from build123d import *

# Parameters (mm, degrees)
F0_W     = 30
F0_H     = 12
F1_DEPTH = 4.5
F2_W     = 30
F2_H     = 12
F3_DEPTH = 30


with BuildPart() as f1:
    # F0 (on Front) → F1 (new body, symmetric)
    with BuildSketch(Plane.XZ):
        with BuildLine():
            Line((8.60261, 24.451202), (-2.39739, 24.451202))
            ThreePointArc((-2.39739, 24.451202), (-9.114904, 21.668717), (-11.89739, 14.951202))
            Line((-11.89739, 14.951202), (-11.89739, -3.548798))
            Line((-11.89739, -3.548798), (18.10261, -3.548798))
            Line((18.10261, -3.548798), (18.10261, 14.951202))
            ThreePointArc((18.10261, 14.951202), (15.320125, 21.668717), (8.60261, 24.451202))
        make_face()
        with Locations((3.10261, -9.548798)):
            Rectangle(F0_W, F0_H)
    extrude(amount=F1_DEPTH, both=True)

    # F2 (on Front) → F3 (join)
    with BuildSketch(Plane.XZ):
        with Locations((3.045083, -9.593663)):
            Rectangle(F2_W, F2_H)
    extrude(amount=F3_DEPTH)


solid = f1.part
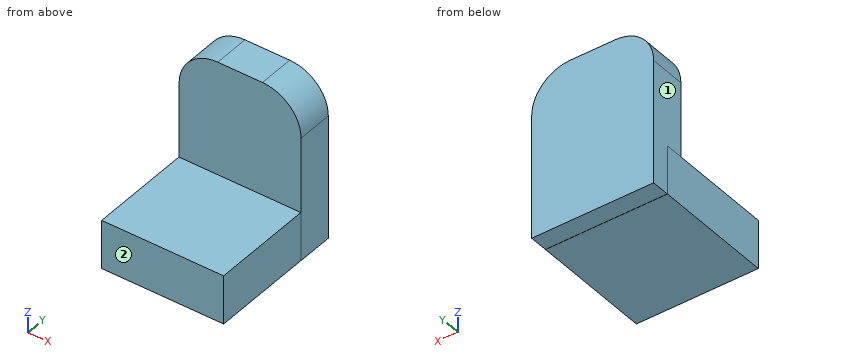
Verification items for the finished model (mm, model axes). Face numbers are marked on the shaded views. A direction names the side the tool comes from. Round coordinates to 2 decimals unless told otherwise and drop trailing zeros. Loops run counter-clockwise (first coordinate to the right, second up) from the corner with the lowest first, then second, coordinate; pieces in that order, holes last. Notation, with made-up numbers: (75.25, 45.25) - (90.25, 45.25) arc R16 cw to (90.25, 61.25) - close; hole circle Ø5 at (71, -19). An arc over 180 degrees is marked (long way). Answer in a Markdown table with one row per item. Add a question column.
Q1. Tool access check on the marked faces 1 and 2. Record the directions out of +Z, -Z, +X, -X, +Y, -Y that give a thin tool (end or side, any length) a straight path to the whole face; none if there is none.
Q2. Section check C-C on z = 8.5. Enter the section's corners in (x, y).
Q3. Gauge pin test, flat ends, axial feed: pin 1 (9.5 mm diameter, centred on y = -20.5, z = -10, fed in from +X); pin 2 (4 mm diameter, centred on x = -4.5, z = 4.5, fed in from -Y); pin 3 (2.5 mm diameter, centred on y = 2, z = 2.5, fed in from -X). Record the tip position at first contact, or that the pin passes through.
Q4. Section check B-B on x = 0. Enter the section's corners in (y, z), plus the area to 3 significant figures.
Q5. Section check D-D on y = 1. Enter the section's corners in (x, z).
Q6. Section check A-A on y = -4. Enter the section's corners in (x, z), plus the area to 3 significant figures.
Q7. Material ranges on line 1 (Z direction, x = -2, y = 2); line 2 (Y direction, x = 13, z = 21); line 3 (Z direction, x = 9, y = -13.5), recorded low to high.
Found:
| question | item | result |
|---|---|---|
| 1 | face 1 | +Z, -X, +Y |
| 1 | face 2 | +Z, -Z, +X, -X, -Y |
| 2 | outline | (-11.9, -4.5) - (18.1, -4.5) - (18.1, 4.5) - (-11.9, 4.5) - close |
| 3 | pin 1 | stops at x = 18.05 |
| 3 | pin 2 | stops at y = -4.5 |
| 3 | pin 3 | stops at x = -11.9 |
| 4 | outline | (-30, -15.59) - (0, -15.59) - (0, -15.55) - (4.5, -15.55) - (4.5, 24.45) - (-4.5, 24.45) - (-4.5, -3.59) - (-30, -3.59) - close |
| 4 | area | 666 mm² |
| 5 | outline | (-11.9, -15.55) - (18.1, -15.55) - (18.1, 14.95) arc R9.5 ccw to (8.6, 24.45) - (-2.4, 24.45) arc R9.5 ccw to (-11.9, 14.95) - close |
| 6 | outline | (-11.95, -15.59) - (18.05, -15.59) - (18.05, -15.55) - (18.1, -15.55) - (18.1, 14.95) arc R9.5 ccw to (8.6, 24.45) - (-2.4, 24.45) arc R9.5 ccw to (-11.9, 14.95) - (-11.9, -3.59) - (-11.95, -3.59) - close |
| 6 | area | 1,160 mm² |
| 7 | line 1 | z = -15.55 to 24.45 |
| 7 | line 2 | y = -4.5 to 4.5 |
| 7 | line 3 | z = -15.59 to -3.59 |
